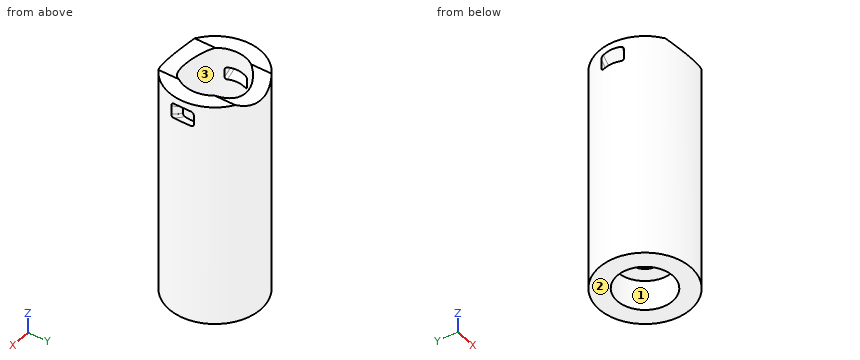
```python
from build123d import *

# Parameters (mm, degrees)
SKETCH1_R               = 6.1
SKETCH1_R_2             = 1.65
BOSS_EXTRUDE1_DEPTH     = 30
SKETCH2_R               = 3.69
CUT_EXTRUDE1_DEPTH      = 4
SKETCH3_R               = 4.09
CUT_EXTRUDE3_DEPTH      = 22
CUT_EXTRUDE4_DEPTH      = 32.215701177
CUT_EXTRUDE4_DEPTH_BACK = 32.215701177
SKETCH4_R               = 6


with BuildPart() as part:
    # Sketch1 → Boss-Extrude1 (new body)
    with BuildSketch(Plane.XY):
        Circle(SKETCH1_R)
        Circle(SKETCH1_R_2, mode=Mode.SUBTRACT)
    extrude(amount=BOSS_EXTRUDE1_DEPTH)

    # Sketch2 → Cut-Extrude1 (cut)
    with BuildSketch(Plane(origin=(0, 0, 0), x_dir=(-1, 0, 0), z_dir=(0, 0, -1))):
        Circle(SKETCH2_R)
    extrude(amount=-CUT_EXTRUDE1_DEPTH, mode=Mode.SUBTRACT)

    # Sketch3 → Cut-Extrude3 (cut)
    with BuildSketch(Plane.XY.offset(30)):
        Circle(SKETCH3_R)
    extrude(amount=-CUT_EXTRUDE3_DEPTH, mode=Mode.SUBTRACT)

    # Sketch4 → Cut-Extrude4 (cut, two sides: drawn at the far end of the back side and taken through both)
    with BuildSketch(Plane(origin=(0, 0, 0), x_dir=(1, 0, 0), z_dir=(0, 1, 0)).offset(-CUT_EXTRUDE4_DEPTH_BACK)):
        with Locations((0, -35)):
            Circle(SKETCH4_R)
    extrude(amount=CUT_EXTRUDE4_DEPTH + CUT_EXTRUDE4_DEPTH_BACK, mode=Mode.SUBTRACT)

    # Sketch7 → Cut-Revolve1 (revolve, cut)
    with BuildSketch(Plane.XY.offset(35)):
        with BuildLine():
            Line((-9.7, 1.5), (-8.8, 1.5))
            ThreePointArc((-8.8, 1.5), (-8.587867966, 1.412132034), (-8.5, 1.2))
            Line((-8.5, 1.2), (-8.5, -1.2))
            ThreePointArc((-8.5, -1.2), (-8.587867966, -1.412132034), (-8.8, -1.5))
            Line((-8.8, -1.5), (-9.7, -1.5))
            ThreePointArc((-9.7, -1.5), (-9.912132034, -1.412132034), (-10, -1.2))
            Line((-10, -1.2), (-10, 1.2))
            ThreePointArc((-10, 1.2), (-9.912132034, 1.412132034), (-9.7, 1.5))
        make_face()
    revolve(axis=Axis((0, 6.1, 35), (0, -1, 0)), mode=Mode.SUBTRACT)


solid = part.part
```
Could you check a few things on this model? Use its own coordinates, in mm. Face numbers are marked on the shaded views. A direction names the side the tool comes from. Round coordinates to 2 decimals unless told otherwise and drop trailing zeros. Write each loop counter-clockwise with the first axis right and the second up, starting at its lowest first coordinate (ties: lowest second). Pieces come first, ordered by that corner, then holes. Notation, with made-up numbers: M 43,56.5 L 71,56.5 A7 ccw 71,69.5 Z; hole C 80.25,-36 d11. An arc over 180 degrees is marked long. Answer in a Markdown table with one row per item. Add a question column.
Q1. Imagine slicing it at A-A (x = 0). Please give me the cut outline in (y, z), then the cut area to 3 significant figures.
Q2. Imagine slicing it at B-B (y = 0). Please give me the cut outline in (x, z), then the cut area to 3 significant figures.
Q3. Will these pins go through, and if not, where does the flat tip stop? pin 1 Ø0.6 at (x, z) = (4.5, 28) entering from -Y; pin 2 Ø5 at (x, y) = (0, 0) entering from -Z; pin 3 Ø4 at (x, y) = (1.5, 0) entering from +Z.
Q4. Imagine slicing it at C-C (z = 19). Please give me the cut outline in (x, y), then the cut area to 3 significant figures.
Q5. If I drill on line 1 (X direction, y = 0, z = 5.2); line 2 (X direction, y = 0, z = 15.5); line 3 (Z direction, x = -3.75, y = -1.5), over which ranges is the centre line in solid material (lowest first)? Write a range as from..to.
Q6. On a 3-axis mill with a long thin cutter (end or side, diameter ignored), from which of +Z, -Z, +X, -X, +Y, -Y can I reach the whole of each face in a straight line? I mean the marked faces 1, 2 and 3. Say none if no direction works.
Q7. Imagine slicing it at D-D (x = 2). Please give me the cut outline in (y, z).
Values:
| question | item | result |
|---|---|---|
| 1 | outline | M -6.1,0 L -3.69,0 L -3.69,4 L -1.65,4 L -1.65,8 L -4.09,8 L -4.09,29 L -6.1,29 Z; M 1.65,4 L 3.69,4 L 3.69,0 L 6.1,0 L 6.1,29 L 4.09,29 L 4.09,8 L 1.65,8 Z |
| 1 | area | 139 mm^2 |
| 2 | outline | M -6.1,0 L -3.69,0 L -3.69,4 L -1.65,4 L -1.65,8 L -4.09,8 L -4.09,25.87 A10 cw -6.1,27.08 Z; M -6.1,29.08 A8.5 ccw -4.09,27.55 L -4.09,30 L -6.1,30 Z; M 1.65,4 L 3.69,4 L 3.69,0 L 6.1,0 L 6.1,27.08 A10 cw 4.09,25.87 L 4.09,8 L 1.65,8 Z; M 4.09,27.55 A8.5 ccw 6.1,29.08 L 6.1,30 L 4.09,30 Z |
| 2 | area | 136 mm^2 |
| 3 | pin 1 | y = -4.42 |
| 3 | pin 2 | z = 4 |
| 3 | pin 3 | z = 8 |
| 4 | outline | C 0,0 d12.2; hole C 0,0 d8.18 |
| 4 | area | 64.3 mm^2 |
| 5 | line 1 | -6.1..-1.65, 1.65..6.1 |
| 5 | line 2 | -6.1..-4.09, 4.09..6.1 |
| 5 | line 3 | 0..8 |
| 6 | face 1 | -Z |
| 6 | face 2 | -Z, +X, -X, +Y, -Y |
| 6 | face 3 | +Z |
| 7 | outline | M -5.76,0 L -3.1,0 L -3.1,4 L 3.1,4 L 3.1,0 L 5.76,0 L 5.76,29.34 L 3.57,29.34 L 3.57,8 L -3.57,8 L -3.57,29.34 L -5.76,29.34 Z |
